from build123d import *

# Parameters (mm, degrees)
SKETCH1_R           = 1.55
SKETCH1_R_2         = 4.25
SKETCH1_R_3         = 1.1
BOSS_EXTRUDE1_DEPTH = 5
SKETCH2_R           = 11.5
CUT_EXTRUDE1_DEPTH  = 1.75
CUT_EXTRUDE2_DEPTH  = 3
SKETCH5_R           = 8
SKETCH5_R_2         = 1.55
BOSS_EXTRUDE2_DEPTH = 3
FILLET1_R           = 1


with BuildPart() as part:
    # Sketch1 → Boss-Extrude1 (new body)
    with BuildSketch(Plane.XY):
        with BuildLine():
            Line((-22.926334266, 5.526262294), (-25.904655941, -19.113737706))
            ThreePointArc((-25.904655941, -19.113737706), (-14.984143133, -31.433737706), (-4.063630324, -19.113737706))
            Line((-4.063630324, -19.113737706), (-7.041951999, 5.526262294))
            ThreePointArc((-7.041951999, 5.526262294), (-14.984143133, 12.566262294), (-22.926334266, 5.526262294))
        make_face()
        with Locations((-14.984143133, 4.566262294)):
            Circle(SKETCH1_R, mode=Mode.SUBTRACT)
        with Locations((-14.984143133, -20.433737706)):
            Circle(SKETCH1_R_2, mode=Mode.SUBTRACT)
        with Locations((-6.984143133, -20.433737706)):
            Circle(SKETCH1_R_3, mode=Mode.SUBTRACT)
        with Locations((-9.327288883, -26.090591955)):
            Circle(SKETCH1_R_3, mode=Mode.SUBTRACT)
        with Locations((-14.984143133, -28.433737706)):
            Circle(SKETCH1_R_3, mode=Mode.SUBTRACT)
        with Locations((-20.640997382, -26.090591955)):
            Circle(SKETCH1_R_3, mode=Mode.SUBTRACT)
        with Locations((-22.984143133, -20.433737706)):
            Circle(SKETCH1_R_3, mode=Mode.SUBTRACT)
        with Locations((-20.640997382, -14.776883456)):
            Circle(SKETCH1_R_3, mode=Mode.SUBTRACT)
        with Locations((-14.984143133, -12.433737706)):
            Circle(SKETCH1_R_3, mode=Mode.SUBTRACT)
        with Locations((-9.327288883, -14.776883456)):
            Circle(SKETCH1_R_3, mode=Mode.SUBTRACT)
    extrude(amount=BOSS_EXTRUDE1_DEPTH)

    # Sketch2 → Cut-Extrude1 (cut)
    with BuildSketch(Plane.XY.offset(5)):
        with Locations((-14.984143133, -20.433737706)):
            Circle(SKETCH2_R)
    extrude(amount=-CUT_EXTRUDE1_DEPTH, mode=Mode.SUBTRACT)

    # Sketch3 → Cut-Extrude2 (cut)
    with BuildSketch(Plane.XY):
        Polygon((-15.415032752, 7.712318154), (-17.924152238, 5.766128868), (-17.493262619, 2.620073008), (-14.553253513, 1.420206435), (-12.044134027, 3.366395721), (-12.475023646, 6.512451581), align=None)
    extrude(amount=CUT_EXTRUDE2_DEPTH, mode=Mode.SUBTRACT)

    # Sketch5 → Boss-Extrude2 (add)
    with BuildSketch(Plane.XY.offset(5)):
        with Locations(Location((-14.88966218, 3.876428191, 0), (0, 0, 9.899538967))):
            Circle(SKETCH5_R)
        with Locations(Location((-14.88966218, 3.876428191, 0), (0, 0, 174.819185621))):
            Circle(SKETCH5_R_2, mode=Mode.SUBTRACT)
    extrude(amount=BOSS_EXTRUDE2_DEPTH)

    # Fillet1
    # the kernel refuses this fillet: 1 mm, written as the material it takes off along each edge
    with BuildSketch(Plane(origin=(-4.063630324, -19.113737706, 0), x_dir=(-0.9927738916792687, -0.11999999999999997, 0), z_dir=(-0.11999999999999997, 0.9927738916792685, 0))) as fillet1_piece_1:
        with BuildLine():
            CenterArc((FILLET1_R, FILLET1_R), FILLET1_R, 180, 90)
            Line((0, FILLET1_R), (0, 0))
            Line((0, 0), (FILLET1_R, 0))
        make_face()
    extrude(amount=24.819347292, mode=Mode.SUBTRACT)
    with BuildSketch(Plane(origin=(-14.984143133, -20.433737706, 0), x_dir=(-0.9927738916792687, 0.1199999999999997, 0), z_dir=(0.1199999999999997, 0.9927738916792687, 0))) as fillet1_piece_2:
        with BuildLine():
            CenterArc((11 - FILLET1_R, FILLET1_R), FILLET1_R, 270, 90)
            Line((11, FILLET1_R), (11, 0))
            Line((11, 0), (11 - FILLET1_R, 0))
        make_face()
    revolve(axis=Axis((-14.984143133, -20.433737706, 0), (0, 0, 1)), revolution_arc=193.784205159, mode=Mode.SUBTRACT)
    with BuildSketch(Plane(origin=(-14.984143133, -20.433737706, 5), x_dir=(0.980329402644487, 0.19736834171341458, 0), z_dir=(0.19736834171341458, -0.980329402644487, 0))) as fillet1_piece_3:
        with BuildLine():
            CenterArc((11.5 + FILLET1_R, -FILLET1_R), FILLET1_R, 90, 90)
            Line((11.5 + FILLET1_R, 0), (11.5, 0))
            Line((11.5, 0), (11.5, -FILLET1_R))
        make_face()
    revolve(axis=Axis((-14.984143133, -20.433737706, 5), (0, 0, 1)), revolution_arc=157.233782309, mode=Mode.SUBTRACT)
    with BuildSketch(Plane(origin=(-14.984143133, 4.566262294, 0), x_dir=(0.9927738916792685, 0.12000000000000052, 0), z_dir=(0.12000000000000052, -0.9927738916792685, 0))) as fillet1_piece_4:
        with BuildLine():
            CenterArc((8 - FILLET1_R, FILLET1_R), FILLET1_R, 270, 90)
            Line((8, FILLET1_R), (8, 0))
            Line((8, 0), (8 - FILLET1_R, 0))
        make_face()
    revolve(axis=Axis((-14.984143133, 4.566262294, 0), (0, 0, 1)), revolution_arc=166.215794841, mode=Mode.SUBTRACT)
    with BuildSketch(Plane(origin=(-22.926334266, 5.526262294, 0), x_dir=(0, 0, 1), z_dir=(-0.11999999999999994, -0.9927738916792685, 0))) as fillet1_piece_5:
        with BuildLine():
            CenterArc((FILLET1_R, -FILLET1_R), FILLET1_R, 90, 90)
            Line((0, -FILLET1_R), (0, 0))
            Line((0, 0), (FILLET1_R, 0))
        make_face()
    extrude(amount=24.819347292, mode=Mode.SUBTRACT)
    with BuildSketch(Plane(origin=(-4.16612256, -18.265807573, 5), x_dir=(-0.9927738916792687, -0.11999999999999998, 0), z_dir=(-0.11999999999999997, 0.9927738916792685, 0))) as fillet1_piece_6_section:
        with BuildLine():
            CenterArc((FILLET1_R, -FILLET1_R), FILLET1_R, 90, 90)
            Line((0, -FILLET1_R), (0, 0))
            Line((0, 0), (FILLET1_R, 0))
        make_face()
    fillet1_piece_6 = extrude(amount=25.349333785, mode=Mode.PRIVATE)
    fillet1_piece_6 = fillet1_piece_6 - Plane(origin=(-14.88966218, 3.876428191, 4.768901456), x_dir=(0.9851107095579202, 0.17192117354849282, 0), z_dir=(0, 0, -1)) * Cylinder(8, 55, mode=Mode.PRIVATE)
    add(fillet1_piece_6, mode=Mode.SUBTRACT)
    with BuildSketch(Plane(origin=(-6.708776504, 2.76986285, 5), x_dir=(-0.9927738916792687, -0.11999999999999998, 0), z_dir=(-0.11999999999999997, 0.9927738916792685, 0))) as fillet1_piece_7_section:
        with BuildLine():
            CenterArc((FILLET1_R, -FILLET1_R), FILLET1_R, 90, 90)
            Line((0, -FILLET1_R), (0, 0))
            Line((0, 0), (FILLET1_R, 0))
        make_face()
    fillet1_piece_7 = extrude(amount=2.776462463, mode=Mode.PRIVATE)
    fillet1_piece_7 = fillet1_piece_7 - Plane(origin=(-14.88966218, 3.876428191, 4.554846091), x_dir=(0.9851107095579202, 0.17192117354849282, 0), z_dir=(0, 0, -1)) * Cylinder(8, 10, mode=Mode.PRIVATE)
    add(fillet1_piece_7, mode=Mode.SUBTRACT)
    with BuildSketch(Plane(origin=(-22.926334266, 5.526262294, 5), x_dir=(0, 0, -1), z_dir=(-0.11999999999999994, -0.9927738916792685, 0))) as fillet1_piece_8_section:
        with BuildLine():
            CenterArc((FILLET1_R, FILLET1_R), FILLET1_R, 180, 90)
            Line((0, FILLET1_R), (0, 0))
            Line((0, 0), (FILLET1_R, 0))
        make_face()
    fillet1_piece_8 = extrude(amount=23.965245326, mode=Mode.PRIVATE)
    fillet1_piece_8 = fillet1_piece_8 - Plane(origin=(-14.88966218, 3.876428191, 4.768639771), x_dir=(0.9851107095579202, 0.17192117354849282, 0), z_dir=(0, 0, -1)) * Cylinder(8, 52, mode=Mode.PRIVATE)
    add(fillet1_piece_8, mode=Mode.SUBTRACT)
    with BuildSketch(Plane(origin=(-14.984143133, 4.566262294, 5), x_dir=(0.9927738916792685, 0.12000000000000052, 0), z_dir=(0.12000000000000052, -0.9927738916792685, 0))) as fillet1_piece_9_section:
        with BuildLine():
            CenterArc((8 - FILLET1_R, -FILLET1_R), FILLET1_R, 0, 90)
            Line((8, -FILLET1_R), (8, 0))
            Line((8, 0), (8 - FILLET1_R, 0))
        make_face()
    fillet1_piece_9 = revolve(axis=Axis((-14.984143133, 4.566262294, 5), (0, 0, 1)), revolution_arc=166.215794841, mode=Mode.PRIVATE)
    fillet1_piece_9 = fillet1_piece_9 - Plane(origin=(-14.88966218, 3.876428191, 4.59944893), x_dir=(0.9851107095579202, 0.17192117354849282, 0), z_dir=(0, 0, -1)) * Cylinder(8, 33, mode=Mode.PRIVATE)
    add(fillet1_piece_9, mode=Mode.SUBTRACT)


solid = part.part
The model under review builds one solid part; all positions refer to its coordinate system, in mm. A direction names the side the tool comes from. Coordinates: 2 decimals unless noted, no trailing zeros. Write each loop counter-clockwise with the first axis right and the second up, starting at its lowest first coordinate (ties: lowest second). Pieces come first, ordered by that corner, then holes. Notation, with made-up numbers: M 57,88 L 104,88 A21 ccw 104,124 Z; hole C 32.25,18.25 d10. An arc over 180 degrees is marked long. Put each result on its own line as item: value.
1) Wall thickness on probe 1 along Z at (x, y) = (-20.75, -8); probe 2 along X at (y, z) = (7.5, 1.5); probe 3 along X at (y, z) = (-13, 3): over which ranges is each line inside the solid? List them lowest first. Write a range as [from, to].
Computed:
probe 1: z = [0, 5]
probe 2: x = [-22.43, -15.69], [-14.89, -7.54]
probe 3: x = [-25.17, -15.93], [-14.04, -4.8]
2) For faces 1 (the cylindrical face through (-21.74, -26.04, 1.6)), 2 (the cylindrical face through (-16.404, 3.546, 6.479)), 3 (the flat face through (-13.924, 7.104, 1.479)), list the 3-axis set-ups (+Z, -Z, +X, -X, +Y, -Y) from which the entire face can be reached by the end or side of a thin tool; tool diameter is ignored.
Computed:
face 1: +Z, -Z
face 2: +Z
face 3: -Z
3) Add section A-A on z = 2. State how many separate pieces and enclosed holes the cut face has, then the cut area to 3 significant figures.
Computed:
separate pieces: 1
enclosed holes: 10
area: 656 mm2
4) Draft analysis for pull direction Y (two halves, no side actions). For faces 4 (the flat face through (-17.712, 4.215, 1.479)), 5 (the flat face through (-15, -25, 3.25)), 6 (the flat face through (-13.316, 2.38, 1.479)), 7 (the cylindrical face through (-14.798, -8.935, 3.63)), state which applies: released by +Y, released by -Y, zero draft, split by the parting line, or undercut.
Computed:
face 4: undercut
face 5: zero draft
face 6: undercut
face 7: released by -Y
5) Clearance check with flat-ended pins moving along their axes: pin 1 Ø1.7 at (x, y) = (-15.5, 5.5) entering from -Z; pin 2 Ø1.5 at (x, z) = (-23, 4.5) entering from -Y; pin 3 Ø6 at (x, y) = (-12, -14.5) entering from -Z; pin 4 Ø2 at (x, z) = (-10.5, 2) entering from +Y. State where each tip first meets the part, or that it passes through.
Computed:
pin 1: stops at z = 3
pin 2: stops at y = -12.89
pin 3: stops at z = 0
pin 4: stops at y = 11.77
6) Add section B-B on z = 6. Give the boundary of the cut face in (x, y), then the cut area to 3 significant figures.
Computed:
outline: C -14.89,3.88 d16; hole C -14.89,3.88 d3.1
area: 194 mm2
